Build history of the part. All positions in model axes, mm. A direction names the side the tool comes from. Give positions to 0.01 mm unless a question says otherwise; leave off trailing zeros. Write each loop counter-clockwise with the first axis right and the second up, starting at its lowest first coordinate (ties: lowest second). Pieces come first, ordered by that corner, then holes.
from build123d import *

# Parameters (mm, degrees)
BASPROSKE_W         = 6.604
BASPROSKE_H         = 10.16
TOOTHCUT_DEPTH      = 16.813412535
TEETHCUTS_COUNT     = 14
TEETHCUTS_ANGLE     = 334.285714286
BORSKE_R            = 4.191
BORE_DEPTH          = 50.8000508
BOSS_EXTRUDE1_START = 1.651
SKETCH1_R           = 5.842
SKETCH1_R_2         = 4.191
BOSS_EXTRUDE1_DEPTH = 1.651
CUT_EXTRUDE1_START  = -8.255
CUT_EXTRUDE1_DEPTH  = 8.255
CHAMFER1_SIZE       = 0.254


# Read off the part's stored shape, not the designer's step: Cut-Extrude1
with BuildPart() as part:
    # BasProSke → Base-Revolve (revolve)
    with BuildSketch(Plane(origin=(0, 0, 0), x_dir=(1, 0, 0), z_dir=(0, 1, 0)), mode=Mode.PRIVATE) as base_revolve_sk:
        with Locations((3.302, 5.08)):
            Rectangle(BASPROSKE_W, BASPROSKE_H)
    revolve(base_revolve_sk.sketch.rotate(Axis((-10, 0, 0), (1, 0, 0)), 180), axis=Axis((-10, 0, 0), (1, 0, 0)))

    # TooCutSke → ToothCut (cut, through all)
    with BuildSketch(Plane(origin=(0, 0, 0), x_dir=(0, 0, -1), z_dir=(1, 0, 0))):
        with BuildLine():
            ThreePointArc((0.690270933, 7.282559789), (0, 7.3152), (-0.690270933, 7.282559789))
            ThreePointArc((-0.690270933, 7.282559789), (-1.062455419, 8.780807329), (-2.034499207, 9.980139585))
            ThreePointArc((-2.034499207, 9.980139585), (0, 10.1854), (2.034499207, 9.980139585))
            ThreePointArc((2.034499207, 9.980139585), (1.062455419, 8.780807329), (0.690270933, 7.282559789))
        make_face()
    toothcut = extrude(amount=TOOTHCUT_DEPTH, mode=Mode.SUBTRACT)

    # TeethCuts: ToothCut ×14 about axis
    teethcuts_axis = Axis((-10, 0, 0), (1, 0, 0))
    for i in range(1, TEETHCUTS_COUNT):
        add(toothcut.rotate(teethcuts_axis, i * TEETHCUTS_ANGLE / (TEETHCUTS_COUNT - 1)), mode=Mode.SUBTRACT)

    # BorSke → Bore (cut, symmetric)
    with BuildSketch(Plane(origin=(0, 0, 0), x_dir=(0, 0, -1), z_dir=(1, 0, 0))):
        with Locations(Location((0, 0, 0), (0, 0, 180))):
            Circle(BORSKE_R)
    extrude(amount=BORE_DEPTH, both=True, mode=Mode.SUBTRACT)

    # Sketch1 → Boss-Extrude1 (add)
    with BuildSketch(Plane(origin=(6.604, 0, 0), x_dir=(0, 0, -1), z_dir=(1, 0, 0)).offset(BOSS_EXTRUDE1_START)):
        with Locations(Location((0, 0, 0), (0, 0, 180))):
            Circle(SKETCH1_R)
        Circle(SKETCH1_R_2, mode=Mode.SUBTRACT)
    extrude(amount=-BOSS_EXTRUDE1_DEPTH)

    # Cut-Extrude1 outline → Cut-Extrude1 (cut)
    with BuildSketch(Plane.ZY.offset(CUT_EXTRUDE1_START)):
        with BuildLine():
            Line((1.105905968, 5.334), (-1.053094032, 5.334))
            Line((-1.053094032, 5.334), (-1.053094032, 4.056534723))
            ThreePointArc((-1.053094032, 4.056534723), (0.02732811, 4.1909109), (1.105905968, 4.042456306))
            Line((1.105905968, 4.042456306), (1.105905968, 5.334))
        make_face()
    extrude(amount=CUT_EXTRUDE1_DEPTH, mode=Mode.SUBTRACT)

    # Chamfer1
    chamfer1_edges = [part.edges().sort_by_distance(p)[0] for p in [
        (8.255, 0, -5.842),
    ]]
    chamfer(chamfer1_edges, length=CHAMFER1_SIZE)


solid = part.part
(1) Drop flat-ended pins along their axis: pin 1 (2 mm diameter, centred on x = 3.5, y = -1.5, fed in from +Z); pin 2 (1.4 mm diameter, centred on x = 5, y = 4.5, fed in from -Z); pin 3 (3 mm diameter, centred on x = 3.5, y = 6.5, fed in from +Z). Give the stop position or say it passes through.
(2) Probe line 1 (Y direction, x = 3, z = 0); line 2 (Y direction, x = 6.25, z = 8.5); line 3 (X direction, y = 0.25, z = 7.25). List the from-to ranges inside material, lowest first.
(3) 3-axis set-ups, long thin cutter, end or side, ignore diameter. For faces 5 (the face through (3.256, -2.993, -8.328)), 6 (the face through (3.256, 2.993, 8.328)), 7 (the face through (7.3, 3.6, -4.6)), 8 (the face through (3.256, -8.377, -2.853)): which of +Z, -Z, +X, -X, +Y, -Y reach the whole face in a straight line?
(4) Mould opens along Y. For faces 1 (the face through (3.26, 4.55, -5.73)), 2 (the face through (3.26, -7.45, 4.77)), 3 (the face through (0, -0.1, -4.4)), 4 (the face through (3.26, 7.45, -4.77)) say: +Y half, -Y half, draft (parallel to the pull), parting line (faces both ways), or undercut.
(5) Saw through at B-B, the plane z = 8. List the corners of the cut face in (x, y).
(6) Saw through at A-A, the plane z = 0. List the corners of the cut face in (x, y) (3 decimals), plus the area to 3 significant figures.
(7) Saw through at C-C, the plane z = -7.5. List the corners of the cut face in (x, y).
Computed values:
1. pin 1: stops at z = 9.81
1. pin 2: stops at z = -9.26
1. pin 3: stops at z = 6.53
2. line 1: y = -7.32 to -4.19, 5.33 to 7.32
2. line 2: y = -4.72 to -3.14, -0.98 to 0.98, 3.14 to 4.72
2. line 3: x = 0 to 6.6
3. face 5: -Z, +X, -X
3. face 6: +Z, +X, -X
3. face 7: +X
3. face 8: +X, -X
4. face 1: undercut
4. face 2: -Y half
4. face 3: draft
4. face 4: +Y half
5. outline: (0, -4.71) - (6.6, -4.71) - (6.6, -2.75) - (0, -2.75) - close; (0, -1.02) - (6.6, -1.02) - (6.6, 1.02) - (0, 1.02) - close; (0, 2.75) - (6.6, 2.75) - (6.6, 4.71) - (0, 4.71) - close
6. outline: (0, -7.315) - (6.604, -7.315) - (6.604, -5.842) - (8.001, -5.842) - (8.255, -5.588) - (8.255, -4.191) - (0, -4.191) - close; (0, 5.334) - (8.255, 5.334) - (8.255, 5.588) - (8.001, 5.842) - (6.604, 5.842) - (6.604, 7.315) - (0, 7.315) - close
6. area: 37.2 mm2
7. outline: (0, -4.64) - (6.6, -4.64) - (6.6, -2.48) - (0, -2.48) - close; (0, -0.99) - (6.6, -0.99) - (6.6, 0.99) - (0, 0.99) - close; (0, 2.48) - (6.6, 2.48) - (6.6, 4.64) - (0, 4.64) - close
